Can you work these out from the drawing? Everything is in mm from the part's minimum corner. A direction names the side the tool comes from. Round coordinates to 2 decimals unless told otherwise and drop trailing zeros. Write each loop counter-clockwise with the first axis right and the second up, starting at its lowest first coordinate (ties: lowest second). Pieces come first, ordered by that corner, then holes. Notation, with made-up numbers: (85, -24.75) - (112, -24.75) arc R6 ccw to (112, -13.75) - close; hole circle Ø7 at (36, 38). An arc over 180 degrees is marked (long way). One line per item, written item: value. Start each with the question number.
(1) Thinking about a two-plate mould opening in X: for the marked faces 4, 5 and 6, which applies, +X half, -X half, draft (parallel to the pull), parting line (faces both ways), or undercut?
(2) I want a section at A-A on x = 3.7. List the corners of the cut face in (y, z) for me, plus the area to 3 significant figures.
(3) I'm going to push flat-ended pins straight in: pin 1 Ø2 at (x, y) = (27, 6) entering from -Z; pin 2 Ø1 at (x, y) = (18, 4.5) entering from +Z; pin 3 Ø1.5 at (y, z) = (8.5, 3) entering from -X. Where does each tip first touch, or does it pass through?
(4) If I drill on L1, parallel to Y at x = 3.7, z = 7.5; L2, parallel to Z at x = 25.5, y = 8.5; L3, parallel to X at y = 4.5, z = 3.5, over which ranges is the centre line in solid material (lowest first)? Write a range as from..to.
(5) On a 3-axis mill with a long thin cutter (end or side, diameter ignored), from which of +Z, -Z, +X, -X, +Y, -Y can I reach the whole of each face in a straight line? I mean the marked faces 1, 2 and 3. Say none if no direction works.
(6) I want a section at C-C on z = 6.75. List the corners of the cut face in (x, y) for me.
(7) I want a section at D-D on y = 8.5. List the corners of the cut face in (x, z) for me.
(8) I want a section at B-B on y = 3. List the corners of the cut face in (x, z) for me, plus the area to 3 significant figures.
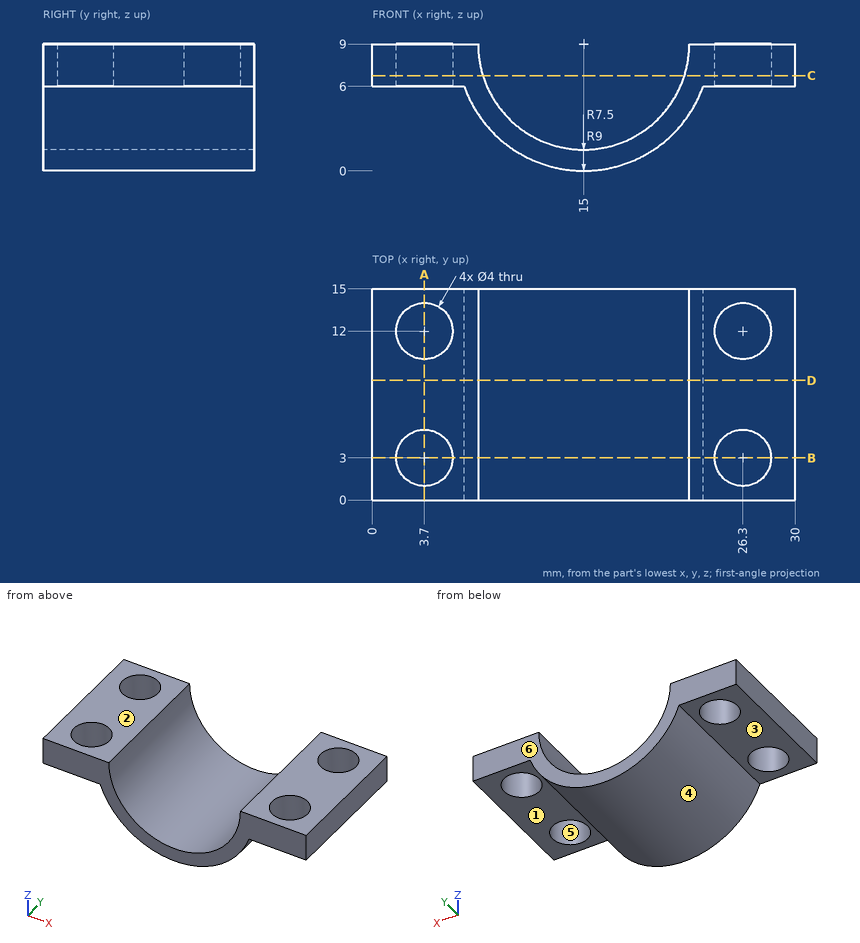
Established:
1. face 4: parting line
1. face 5: undercut
1. face 6: draft
2. outline: (0, 6) - (1, 6) - (1, 9) - (0, 9) - close; (5, 6) - (10, 6) - (10, 9) - (5, 9) - close; (14, 6) - (15, 6) - (15, 9) - (14, 9) - close
2. area: 21.0 mm2
3. pin 1: z = 6
3. pin 2: z = 2.37
3. pin 3: x = 7.69
4. L1: 0..1, 5..10, 14..15
4. L2: 6..9
4. L3: 7.88..9.9, 20.1..22.12
5. face 1: -Z, +X, +Y, -Y
5. face 2: +Z, +X, -X, +Y, -Y
5. face 3: -Z, -X, +Y, -Y
6. outline: (0, 0) - (7.85, 0) - (7.85, 15) - (0, 15) - close; (22.15, 0) - (30, 0) - (30, 15) - (22.15, 15) - close; hole circle Ø4 at (3.7, 3); hole circle Ø4 at (3.7, 12); hole circle Ø4 at (26.3, 3); hole circle Ø4 at (26.3, 12)
7. outline: (0, 6) - (6.51, 6) arc R9 ccw to (23.49, 6) - (30, 6) - (30, 9) - (22.5, 9) arc R7.5 cw to (7.5, 9) - (0, 9) - close
8. outline: (0, 6) - (1.7, 6) - (1.7, 9) - (0, 9) - close; (5.7, 6) - (6.51, 6) arc R9 ccw to (23.49, 6) - (24.3, 6) - (24.3, 9) - (22.5, 9) arc R7.5 cw to (7.5, 9) - (5.7, 9) - close; (28.3, 6) - (30, 6) - (30, 9) - (28.3, 9) - close
8. area: 51.9 mm2
